```python
from build123d import *

# Parameters (mm, degrees)
F0_W     = 32
F0_H     = 50
F1_DEPTH = 5
F3_DEPTH = 5
F4_R     = 1
F5_DEPTH = 2.9
F7_DEPTH = 3


# Not quite as in the source:
# - a pattern or mirror of a feature is missing from the dataset's text; its kind, count and spacing are read off the source's solid


with BuildPart() as f1:
    # F0 (on Top) → F1 (new body)
    with BuildSketch(Plane.XY):
        Rectangle(F0_W, F0_H)
    extrude(amount=F1_DEPTH)

    # F2 (on face) → F3 (cut, through all)
    with BuildSketch(Plane.XY.offset(5)):
        Polygon((11, 25), (-11, 25), (-2.5, 5), (0, 5), (2.5, 5), align=None)
        Polygon((0, -5), (-2.5, -5), (-11, -25), (11, -25), (2.5, -5), align=None)
    extrude(amount=-F3_DEPTH, mode=Mode.SUBTRACT)

    # F4 (on face) → F5 (cut)
    with BuildSketch(Plane(origin=(-16, 0, 0), x_dir=(0, -1, 0), z_dir=(-1, 0, 0))):
        with Locations((-5, 2.5)):
            Circle(F4_R)
        with Locations((5, 2.5)):
            Circle(F4_R)
    f5 = extrude(amount=-F5_DEPTH, mode=Mode.SUBTRACT)

    # F5_copies: F5 across plane
    add(f5.mirror(Plane(origin=(0, 0, 0), x_dir=(0, 0, 1), z_dir=(1, 0, 0))), mode=Mode.SUBTRACT)

    # F6 (on face) → F7 (cut)
    with BuildSketch(Plane.XY.offset(5)):
        Polygon((-11, 25), (-13, 25), (-13, -25), (-11, -25), (-2.5, -5), (2.5, -5), (11, -25), (13, -25), (13, 25), (11, 25), (2.5, 5), (-2.5, 5), align=None)
    extrude(amount=-F7_DEPTH, mode=Mode.SUBTRACT)


solid = f1.part
```
The listing builds one solid part. Answer for the finished solid, in the listing's coordinates (mm). A direction names the side the tool comes from. Give positions to 0.01 mm unless a question says otherwise; leave off trailing zeros. Order: outer loops, then holes, each group sorted by start corner. A loop starts at its lowest first (then second) coordinate and runs counter-clockwise, first axis right, second up. Notation, with made-up numbers: (17, 66) -> (65, 66) arc R21 cw to (65, 105) -> close; hole circle Ø11 at (57, -6.5). An arc over 180 degrees is marked (long way). Answer as CSV lines item,"result". Start each with the question number.
Q1. A cutting plane is placed at B-B (z = 2.5). Determine the outline of the cut face in (x, y).
Q2. A cutting plane is placed at A-A (y = -17). Determine the outline of the cut face in (x, z), then the cut area to 3 significant figures.
Q3. Which of the six approach directions +Z, -Z, +X, -X, +Y, -Y give full straight-line access (tool end or side, diameter ignored) to faces 1 (the cylindrical face through (14.57, -4.87, 3.49)), 2 (the cylindrical face through (-14.57, -4.87, 3.49)), 3 (the flat face through (-6.81, 15.14, 1.01))?
Q4. Find the intervals of material crossed by L1, parallel to X at y = 14, z = 3.1; L2, parallel to Z at x = 10, y = -7; L3, parallel to X at y = -14.5, z = 0.95, in increasing order.
Q5. A cutting plane is placed at D-D (x = 1). Determine the outline of the cut face in (y, z), then the cut area to 3 significant figures.
Q6. A cutting plane is placed at C-C (y = -0.5). Determine the outline of the cut face in (x, z), then the cut area to 3 significant figures.
Q7. Determine the mould class of faces 4 (the flat face through (16, 0, 2)), 5 (the flat face through (13, 0, 4)), 6 (the flat face through (-16, 0, 2)) for opening direction X: pulls with the +X half, pulls with the -X half, needs draft (parallel to the pull), parting line crosses it, or undercut.
Q8. Given pin 1 (1 mm diameter, centred on x = 0.5, z = 0.5, fed in from +Y); pin 2 (1.5 mm diameter, centred on x = -3.5, z = 2, fed in from -Y); pin 3 (1 mm diameter, centred on x = -4, z = 0.5, fed in from -Y), each flat-ended and moving along its own axis, determine where each tip first touches the part or whether it passes through.
Results found:
1,outline,"(-16, -25) -> (-13, -25) -> (-13, 25) -> (-16, 25) -> (-16, 6) -> (-13.1, 6) -> (-13.1, 4) -> (-16, 4) -> (-16, -4) -> (-13.1, -4) -> (-13.1, -6) -> (-16, -6) -> close; (13, -25) -> (16, -25) -> (16, -6) -> (13.1, -6) -> (13.1, -4) -> (16, -4) -> (16, 4) -> (13.1, 4) -> (13.1, 6) -> (16, 6) -> (16, 25) -> (13, 25) -> close"
2,outline,"(-16, 0) -> (-7.6, 0) -> (-7.6, 2) -> (-13, 2) -> (-13, 5) -> (-16, 5) -> close; (7.6, 0) -> (16, 0) -> (16, 5) -> (13, 5) -> (13, 2) -> (7.6, 2) -> close"
2,area,"51.6 mm2"
3,face 1,"+X"
3,face 2,"-X"
3,face 3,"+Z, -Z, +Y"
4,L1,"-16 to -13, 13 to 16"
4,L2,"0 to 2"
4,L3,"-16 to -6.54, 6.54 to 16"
5,outline,"(-5, 0) -> (5, 0) -> (5, 2) -> (-5, 2) -> close"
5,area,"20.0 mm2"
6,outline,"(-16, 0) -> (16, 0) -> (16, 5) -> (13, 5) -> (13, 2) -> (-13, 2) -> (-13, 5) -> (-16, 5) -> close"
6,area,"82.0 mm2"
7,face 4,"pulls with the +X half"
7,face 5,"undercut"
7,face 6,"pulls with the -X half"
8,pin 1,"y = 5"
8,pin 2,"y = -9.12"
8,pin 3,"y = -9.71"
